For this review, take the finished solid that the model builds, in its own axes (mm). A direction names the side the tool comes from. Give positions to 0.01 mm unless a question says otherwise; leave off trailing zeros. Write each loop counter-clockwise with the first axis right and the second up, starting at its lowest first coordinate (ties: lowest second). Pieces come first, ordered by that corner, then holes.
Autodesk Inventor part; units mm, degrees
ref_plane "YZ Plane" through (0, 0, 0) normal (1, 0, 0) x (0, 1, 0)
ref_plane "XZ Plane" through (0, 0, 0) normal (0, 1, 0) x (-1, 0, 0)
ref_plane "XY Plane" through (0, 0, 0) normal (0, 0, 1) x (1, 0, 0)
sketch "スケッチ1" plane through (0, 0, 0) normal (0, 0, 1) x (1, 0, 0)
  line L0 (-60, 10) -> (60, 10)
  line L1 (60, 10) -> (60, -10)
  line L2 (60, -10) -> (-60, -10)
  line L3 (-60, -10) -> (-60, 10)
  line L4 (-60, 10) -> (60, -10) construction
  line L5 (60, 10) -> (-60, -10) construction
  point P0 (0, 0)
  dimension "d0" = 120
  dimension "d1" = 20
extrude "押し出し1" add sketch "スケッチ1" along normal blind 1
sketch "スケッチ2" plane through (0, 0, 1) normal (0, 0, 1) x (1, 0, 0)
  line L0 (60, -10) -> (60, 10)
  line L1 (60, 10) -> (-60, 10)
  line L2 (-60, 10) -> (-60, -10)
  line L3 (-60, -10) -> (60, -10)
  point P0 (0, 0)
  point P1 (14, 5)
  point P2 (14, -5)
  point P3 (45, 0)
  dimension "d4" = 15
  dimension "d5" = 10
  dimension "d7" = 46
  dimension "d8" = 5
  dimension "d9" = 5
hole "穴1" at (14, 5, 1) at (14, -5, 1) at (45, 0, 1) direction (0, 0, -1) diameter 3.2 end through all
sketch "スケッチ3" plane through (0, 0, 1) normal (0, 0, 1) x (1, 0, 0)
  line L0 (-60, 10) -> (-61, 10)
  line L1 (-61, 10) -> (-61, -10)
  line L2 (-61, -10) -> (-60, -10)
  line L3 (-60, -10) -> (-60, 10)
  point P0 (0, 0)
  dimension "d17" = 1
  dimension "d18" = 20
extrude "押し出し2" add sketch "スケッチ3" against normal blind 11
sketch "スケッチ4" plane through (-60, -10, 0) normal (1, 0, 0) x (0, 0, -1)
  line L0 (10, 20) -> (10, 0)
  line L1 (0, 20) -> (10, 20)
  line L2 (0, 0) -> (10, 0)
  point P0 (0, 10)
  point P1 (5, 15)
  point P2 (5, 5)
  dimension "d21" = 5
  dimension "d22" = 5
  dimension "d30" = 5
  dimension "d31" = 5
  dimension "d32" = 10
hole "穴2" at (-60, 5, -5) at (-60, -5, -5) direction (-1, 0, 0) diameter 3.2 end through all
sketch "スケッチ5" plane through (0, 0, 1) normal (0, 0, 1) x (1, 0, 0)
  line L0 (-61, -10) -> (60, -10)
  line L1 (60, 10) -> (50, 10)
  line L2 (50, 10) -> (50, -10)
  line L3 (50, -10) -> (60, -10)
  line L4 (60, -10) -> (60, 10)
  point P0 (0, 0)
  dimension "d33" = 10
extrude "押し出し3" cut sketch "スケッチ5" against normal blind 10
properties part number "爪＿2" material "アルミニウム 6061"
(1) We need section B-B (z = -5). Write out the cut boundary in (x, y).
(2) For L1, parallel to Y at x = -60.55, z = -5; L2, parallel to X at y = 0, z = 0.55; L3, parallel to X at y = -5, z = 0.4, list the stretches that pass through material, from the lowest coordinate up.
(3) Tool access review of faces 4 (the flat face through (-5.2, 10, 0.4)), 5 (the flat face through (-6, 0, 0)): name each direction out of +Z, -Z, +X, -X, +Y, -Y from which nothing blocks a thin tool from reaching the whole face with its end or side.
(4) The part is to be moulded in two halves that separate along Z. For faces 1 (the cylindrical face through (-60.51, -3.44, -4.65)), 2 (the flat face through (-6, 0, 1)), 3 (the flat face through (-60, 0, -5)), say which applies: +Z half, -Z half, draft (parallel to the pull), parting line (faces both ways), or undercut.
(5) We need section D-D (y = -5). Write out the cut boundary in (x, z).
(6) We need section A-A (x = 45). Write out the cut boundary in (y, z).
(7) Clearance check with flat-ended pins moving along their axes: pin 1 Ø1.9 at (x, y) = (14, 5) entering from +Z; pin 2 Ø3.5 at (x, y) = (14, -5) entering from -Z; pin 3 Ø2 at (y, z) = (7, -5.5) entering from +X. State where each tip first meets the part, or that it passes through.
(8) We need section C-C (y = 0). Write out the cut boundary in (x, z).
The answers:
1. outline: (-61, -10) - (-60, -10) - (-60, -6.6) - (-61, -6.6) - close; (-61, -3.4) - (-60, -3.4) - (-60, 3.4) - (-61, 3.4) - close; (-61, 6.6) - (-60, 6.6) - (-60, 10) - (-61, 10) - close
2. L1: y = -10 to -6.6, -3.4 to 3.4, 6.6 to 10
2. L2: x = -61 to 43.4, 46.6 to 50
2. L3: x = -61 to 12.4, 15.6 to 50
3. face 4: +Z, -Z, +X, -X, +Y
3. face 5: -Z, +X, +Y, -Y
4. face 1: undercut
4. face 2: +Z half
4. face 3: draft
5. outline: (-61, -10) - (-60, -10) - (-60, -6.6) - (-61, -6.6) - close; (-61, -3.4) - (-60, -3.4) - (-60, 0) - (12.4, 0) - (12.4, 1) - (-61, 1) - close; (15.6, 0) - (50, 0) - (50, 1) - (15.6, 1) - close
6. outline: (-10, 0) - (-1.6, 0) - (-1.6, 1) - (-10, 1) - close; (1.6, 0) - (10, 0) - (10, 1) - (1.6, 1) - close
7. pin 1: passes through
7. pin 2: stops at z = 0
7. pin 3: stops at x = -60
8. outline: (-61, -10) - (-60, -10) - (-60, 0) - (43.4, 0) - (43.4, 1) - (-61, 1) - close; (46.6, 0) - (50, 0) - (50, 1) - (46.6, 1) - close
